The model under review builds one solid part; all positions refer to its coordinate system, in mm. Coordinates: 2 decimals unless noted, no trailing zeros. Write each loop counter-clockwise with the first axis right and the second up, starting at its lowest first coordinate (ties: lowest second). Pieces come first, ordered by that corner, then holes. Notation, with made-up numbers: (59.5, 20) -> (68.5, 20) arc R27 cw to (68.5, 48) -> close; hole circle Ø4 at (-2, 9). An arc over 180 degrees is marked (long way). Write each question's results on one line, items separated by ' | '.
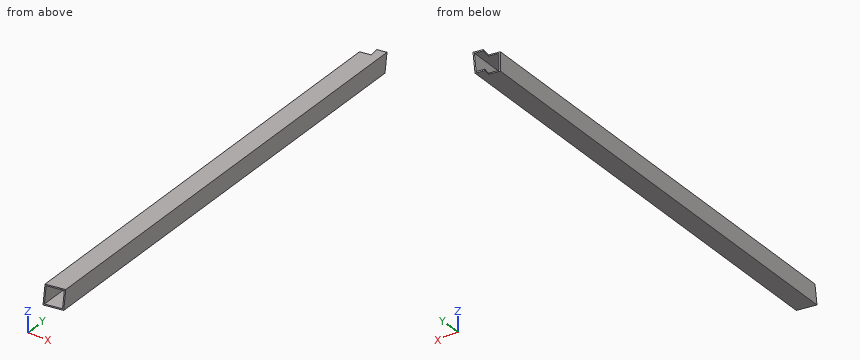
Autodesk Inventor part; units mm, degrees
ref_plane "YZ Plane" through (0, 0, 0) normal (1, 0, 0) x (0, 1, 0)
ref_plane "XZ Plane" through (0, 0, 0) normal (0, 1, 0) x (-1, 0, 0)
ref_plane "XY Plane" through (0, 0, 0) normal (0, 0, 1) x (1, 0, 0)
sketch "Sketch1" plane through (0, 0, 0) normal (0, 1, 0) x (-1, 0, 0)
  line L0 (0, 0) -> (-25.4, 0)
  line L1 (-25.4, 0) -> (-25.4, 25.4)
  line L2 (-25.4, 25.4) -> (0, 25.4)
  line L3 (0, 25.4) -> (0, 0)
  line L4 (-1.5875, 23.8125) -> (-23.8125, 23.8125)
  line L5 (-23.8125, 23.8125) -> (-23.8125, 1.5875)
  line L6 (-23.8125, 1.5875) -> (-1.5875, 1.5875)
  line L7 (-1.5875, 1.5875) -> (-1.5875, 23.8125)
  dimension "d0" = 25.4
  dimension "d2" = 25.4
  dimension "d3" = 1.5875
extrude "Extrusion1" add sketch "Sketch1" along normal blind 1016
ref_plane "Work Plane1" through (102.0769, 3.5287, 0.7496) normal (0.0123, -0.1468, -0.9891) x (-0.1571, 0.9766, -0.1469)
sketch "Sketch4" plane through (102.0769, 3.5287, 0.7496) normal (0.0123, -0.1468, -0.9891) x (-0.1571, 0.9766, -0.1469)
  line L0 (12.7, -101.348) -> (12.7, -75.0726)
  line L1 (12.7, -75.0726) -> (-1.1984, -75.0726)
  line L2 (-1.1984, -75.0726) -> (-1.1984, -113.5605)
  line L3 (-1.1984, -113.5605) -> (12.7, -101.348)
extrude "Extrusion3" cut sketch "Sketch4" along normal mid plane 2540
ref_plane "Work Plane2" through (2.7066, 641.7405, 200.1131) normal (-0.1571, 0.9766, -0.1469) x (0.9875, 0.1572, -0.011)
sketch "Sketch5" plane through (2.7066, 641.7405, 200.1131) normal (-0.1571, 0.9766, -0.1469) x (0.9875, 0.1572, -0.011)
  line L0 (-64.0002, -43.7034) -> (-64.0002, 400.9318)
  line L1 (-64.0002, 400.9318) -> (260.4368, 400.9318)
  line L2 (260.4368, 400.9318) -> (260.4368, -43.7034)
  line L3 (260.4368, -43.7034) -> (-64.0002, -43.7034)
  point P0 (-101.348, 292.1)
extrude "Extrusion4" cut sketch "Sketch5" along normal blind 2540
sketch "Sketch6" plane through (0, 3.8207, 25.4) normal (0, 0, 1) x (1, 0, 0)
  line L0 (25.4, 615.2901) -> (0, 611.2042)
  line L1 (0, 0) -> (0, 611.2042)
  line L2 (0, 0) -> (25.4, 4.0859)
  line L3 (12.7, 613.2471) -> (14.717, 600.7083)
  line L4 (14.717, 600.7083) -> (0, 598.3409)
  point P0 (0, -3.8207)
  dimension "d12" = 12.7
extrude "Extrusion5" cut sketch "Sketch6" against normal blind 25.4
properties part number "Square Tube 4"
Q1. For line 1 (Z direction, x = 21.5, y = 522); line 2 (Y direction, x = 9, z = 1.25), list the stretches that pass through material, from the lowest coordinate up. Write a range as from..to.
Solution:
line 1: 0..1.59, 23.81..25.4 | line 2: 1.64..603.61
Q2. Add section C-C (x = 8). Write out the cut boundary in (y, z), plus the area to 3 significant figures.
Solution:
outline: (1.29, 0) -> (603.45, 0) -> (603.45, 1.59) -> (1.53, 1.59) -> close; (4.87, 23.81) -> (603.45, 23.81) -> (603.45, 25.4) -> (5.11, 25.4) -> close | area: 1,910 mm²
Q3. Add section B-B (y = 187.5). Write out the cut boundary in (x, z), plus the area to 3 significant figures.
Solution:
outline: (0, 0) -> (25.4, 0) -> (25.4, 25.4) -> (0, 25.4) -> close; hole (1.59, 1.59) -> (23.81, 1.59) -> (23.81, 23.81) -> (1.59, 23.81) -> close | area: 151 mm²
Q4. Add section A-A (z = 6). Write out the cut boundary in (x, y), plus the area to 3 significant figures.
Solution:
outline: (0, 0.9) -> (1.59, 1.16) -> (1.59, 602.42) -> (0, 602.16) -> close; (23.81, 4.73) -> (25.4, 4.99) -> (25.4, 616.19) -> (23.81, 615.94) -> close | area: 1,920 mm²
